```python
from build123d import *

# Parameters (mm, degrees)
BOSS_EXTRUDE1_DEPTH          = 5
M3_CLEARANCE_HOLE1_D         = 3.4
M3X0_5_TAPPED_HOLE1_D        = 2.5
M3X0_5_TAPPED_HOLE1_DEPTH    = 7.5
M3X0_5_TAPPED_HOLE1_TIP      = 0.751075774
F_3_0MM_DOWEL_HOLE1_D        = 3
F_3_0MM_DOWEL_HOLE1_DEPTH    = 6
F_3_0MM_DOWEL_HOLE1_TIP      = 0.901290929
M3X0_5_TAPPED_HOLE2_D        = 2.5
M3X0_5_TAPPED_HOLE2_DEPTH    = 7.5
M3X0_5_TAPPED_HOLE2_TIP      = 0.751075774
M6X1_0_TAPPED_HOLE1_D        = 5
M6_CLEARANCE_HOLE1_D         = 6.6
F_7_16_20_TAPPED_HOLE1_D     = 9.92124
F_7_16_20_TAPPED_HOLE1_DEPTH = 17
F_7_16_20_TAPPED_HOLE1_TIP   = 2.980641204


with BuildPart() as part:
    # Sketch1 → Boss-Extrude1 (new, symmetric)
    with BuildSketch(Plane(origin=(0, 0, 0), x_dir=(1, 0, 0), z_dir=(0, 1, 0))):
        Polygon((-131.979797464, 264), (131.979797464, 264), (264, 131.979797464), (264, -131.979797464), (131.979797464, -264), (-131.979797464, -264), (-264, -131.979797464), (-264, 131.979797464), align=None)
    extrude(amount=BOSS_EXTRUDE1_DEPTH, both=True)

    # M3 Clearance Hole1 (through all)
    with Locations(Plane(origin=(0, 5, 0), x_dir=(1, 0, 0), z_dir=(0, 1, 0))):
        with Locations((250.5, 0), (245.686712741, -48.870125665), (231.431822894, -95.862199807), (208.283137882, -139.170343371), (177.130248687, -177.130248687), (139.170343371, -208.283137882), (95.862199807, -231.431822894), (48.870125665, -245.686712741), (0, -250.5), (-48.870125665, -245.686712741), (-95.862199807, -231.431822894), (-139.170343371, -208.283137882), (-177.130248687, -177.130248687), (-208.283137882, -139.170343371), (-231.431822894, -95.862199807), (-245.686712741, -48.870125665), (-250.5, 0), (-245.686712741, 48.870125665), (-231.431822894, 95.862199807), (-208.283137882, 139.170343371), (-177.130248687, 177.130248687), (-139.170343371, 208.283137882), (-95.862199807, 231.431822894), (-48.870125665, 245.686712741), (0, 250.5), (48.870125665, 245.686712741), (95.862199807, 231.431822894), (139.170343371, 208.283137882), (177.130248687, 177.130248687), (208.283137882, 139.170343371), (231.431822894, 95.862199807), (245.686712741, 48.870125665)):
            Hole(M3_CLEARANCE_HOLE1_D / 2)

    # M3x0.5 Tapped Hole1
    with Locations(Plane(origin=(0, 5, 0), x_dir=(1, 0, 0), z_dir=(0, 1, 0))):
        with Locations((209, 9), (209, -9), (112.294228634, -176.499309391), (96.705771366, -185.499309391), (-96.705771366, -185.499309391), (-112.294228634, -176.499309391), (-209, -9), (-209, 9), (-112.294228634, 176.499309391), (-96.705771366, 185.499309391), (96.705771366, 185.499309391), (112.294228634, 176.499309391)):
            Hole(M3X0_5_TAPPED_HOLE1_D / 2, depth=M3X0_5_TAPPED_HOLE1_DEPTH)
            with Locations((0, 0, -(M3X0_5_TAPPED_HOLE1_DEPTH + M3X0_5_TAPPED_HOLE1_TIP / 2))):  # 118° drill point
                Cone(0, M3X0_5_TAPPED_HOLE1_D / 2, M3X0_5_TAPPED_HOLE1_TIP, mode=Mode.SUBTRACT)

    # Ø3.0mm Dowel Hole1
    with Locations(Plane(origin=(0, 5, 0), x_dir=(1, 0, 0), z_dir=(0, 1, 0))):
        with Locations((201, -9), (-201, 9)):
            Hole(F_3_0MM_DOWEL_HOLE1_D / 2, depth=F_3_0MM_DOWEL_HOLE1_DEPTH)
            with Locations((0, 0, -(F_3_0MM_DOWEL_HOLE1_DEPTH + F_3_0MM_DOWEL_HOLE1_TIP / 2))):  # 118° drill point
                Cone(0, F_3_0MM_DOWEL_HOLE1_D / 2, F_3_0MM_DOWEL_HOLE1_TIP, mode=Mode.SUBTRACT)

    # M3x0.5 Tapped Hole2
    with Locations(Plane(origin=(0, 5, 0), x_dir=(1, 0, 0), z_dir=(0, 1, 0))):
        with Locations((-105, -105), (-35, -105), (105, -105), (-35, -35), (35, -35), (105, -35), (-35, 35), (35, 35), (105, 35), (-35, 105), (35, 105), (105, 105), (-105, -35), (-105, 35), (-105, 105)):
            Hole(M3X0_5_TAPPED_HOLE2_D / 2, depth=M3X0_5_TAPPED_HOLE2_DEPTH)
            with Locations((0, 0, -(M3X0_5_TAPPED_HOLE2_DEPTH + M3X0_5_TAPPED_HOLE2_TIP / 2))):  # 118° drill point
                Cone(0, M3X0_5_TAPPED_HOLE2_D / 2, M3X0_5_TAPPED_HOLE2_TIP, mode=Mode.SUBTRACT)

    # M6x1.0 Tapped Hole1 (through all)
    with Locations(Plane(origin=(0, 5, 0), x_dir=(1, 0, 0), z_dir=(0, 1, 0))):
        with Locations((-193.040151264, -193.040151264), (-193.040151264, 193.040151264), (193.040151264, 193.040151264), (193.040151264, -193.040151264)):
            Hole(M6X1_0_TAPPED_HOLE1_D / 2)

    # M6 Clearance Hole1 (through all)
    with Locations(Plane(origin=(0, 5, 0), x_dir=(1, 0, 0), z_dir=(0, 1, 0))):
        with Locations((-125, -250), (-250, -125), (-125, 250), (-250, 125), (125, -250), (250, -125), (250, 125), (125, 250)):
            Hole(M6_CLEARANCE_HOLE1_D / 2)

    # 7/16-20 Tapped Hole1
    with Locations(Plane(origin=(0, -5, 0), x_dir=(-1, 0, 0), z_dir=(0, -1, 0))):
        with Locations((173.205080757, 100)):
            Hole(F_7_16_20_TAPPED_HOLE1_D / 2, depth=F_7_16_20_TAPPED_HOLE1_DEPTH)
            with Locations((0, 0, -(F_7_16_20_TAPPED_HOLE1_DEPTH + F_7_16_20_TAPPED_HOLE1_TIP / 2))):  # 118° drill point
                Cone(0, F_7_16_20_TAPPED_HOLE1_D / 2, F_7_16_20_TAPPED_HOLE1_TIP, mode=Mode.SUBTRACT)


solid = part.part
```
The listing builds one solid part. Answer for the finished solid, in the listing's coordinates (mm). Round coordinates to 2 decimals unless told otherwise and drop trailing zeros. Put each result on its own line as item: value. Start each with the question number.
(1) Given P1, Ø2, axis at x = -112.29, z = 176.5, coming from the +Y side; P2, Ø1, axis at x = 156, y = 3.5, coming from the +Z side; P3, Ø5, axis at x = 186.5, y = 2, coming from the -Z side, each flat-ended and moving along its own axis, determine where each tip first touches the part or whether it passes through.
(2) Straight lines are drawn through the part: probe 1 along X at (y, z) = (-2.75, -100); probe 2 along Z at (x, y) = (140, 1.25); probe 3 along X at (y, z) = (-2.5, 250). For each, find the intervals that lie inside material, in ascending order. Write a range as from..to.
(3) Find section A-A (y = 1.75). State how many separate pieces and enclosed holes the cut face has, plus the area to 3 significant figures.
Reply:
1. P1: y = -2.65
1. P2: z = 240.48
1. P3: z = -211.98
2. probe 1: -264..-178.17, -168.24..264
2. probe 2: -255.98..-209.77, -206.8..206.8, 209.77..255.98
2. probe 3: -145.98..-128.3, -121.7..-1.62, 1.62..121.7, 128.3..145.98
3. separate pieces: 1
3. enclosed holes: 74
3. area: 243,000 mm^2
